Could you check a few things on this model? Use its own coordinates, in mm. Give positions to 0.01 mm unless a question says otherwise; leave off trailing zeros. Order: outer loops, then holes, each group sorted by start corner. A loop starts at its lowest first (then second) coordinate and runs counter-clockwise, first axis right, second up. Notation, with made-up numbers: (84, 79) -> (136, 79) arc R28 cw to (136, 102) -> close; hole circle Ø11 at (22, 53.5). An arc over 180 degrees is marked (long way). One line per item, written item: value.
```python
from build123d import *

# Parameters (mm, degrees)
F0_R     = 10.579835
F0_R_2   = 8.89
F1_DEPTH = 2.286
F2_R     = 0.762


with BuildPart() as f1:
    # F0 (on Front) → F1 (new body)
    with BuildSketch(Plane.XZ):
        with Locations((-48.006002, 40.996861)):
            Circle(F0_R)
        with Locations((-48.006002, 40.996861)):
            Circle(F0_R_2, mode=Mode.SUBTRACT)
    extrude(amount=F1_DEPTH)

    # F2
    f2_edges = [f1.edges().sort_by_distance(p)[0] for p in [
        (-58.585837, -2.286, 40.996861),
        (-58.585837, 0, 40.996861),
        (-56.896002, 0, 40.996861),
        (-56.896002, -2.286, 40.996861),
    ]]
    fillet(f2_edges, radius=F2_R)


solid = f1.part
```
1) For P1, Ø1, axis at y = -0.5, z = 36.5, coming from the +X side; P2, Ø1.5, axis at x = -51.5, z = 33, coming from the +Y side, each with a flat end and sliding along its axis, tell me the tip position at first contact or that it passes through.
Answer below:
P1: stops at x = -38.23
P2: stops at y = -0.02
2) If I drill on line 1 along X through (y, z) = (-1.4, 41); line 2 along X through (y, z) = (-1.8, 35.5); line 3 along Z through (x, y) = (-55.5, -0.25), over which ranges is the centre line in solid material (lowest first)?
Answer below:
line 1: x = -58.59 to -56.9, -39.12 to -37.43
line 2: x = -56.99 to -55.06, -40.95 to -39.03
line 3: z = 33.81 to 35.86, 46.14 to 48.18
3) Suppose I cut it at A-A, the plane y = -2. Write out the boundary of the cut face in (x, z).
Answer below:
outline: circle Ø20.83 at (-48.01, 41); hole circle Ø18.11 at (-48.01, 41)
4) We'd pull the mould along Z, two halves only. Please class faces 1 (the cylindrical face through (-43.9, -1.14, 33.11)), 2 (the cylindrical face through (-58.576, -1.138, 41.462)): +Z half, -Z half, draft (parallel to the pull), parting line (faces both ways), or undercut.
Answer below:
face 1: undercut
face 2: parting line
5) Suppose I cut it at B-B, the plane y = -0.25. Write out the boundary of the cut face in (x, z).
Answer below:
outline: circle Ø20.76 at (-48.01, 41); hole circle Ø18.18 at (-48.01, 41)
